Autodesk Inventor part; units mm, degrees
ref_plane "YZ Plane" through (0, 0, 0) normal (1, 0, 0) x (0, 1, 0)
ref_plane "XZ Plane" through (0, 0, 0) normal (0, 1, 0) x (-1, 0, 0)
ref_plane "XY Plane" through (0, 0, 0) normal (0, 0, 1) x (1, 0, 0)
sketch "Sketch1" plane through (0, 0, 0) normal (1, 0, 0) x (0, 1, 0)
  line L0 (-25, 30) -> (25, 30)
  line L1 (30, 25) -> (30, -25)
  line L2 (25, -30) -> (-25, -30)
  line L3 (-30, -25) -> (-30, 25)
  line L4 (-30, 30) -> (30, -30) construction
  line L5 (30, 30) -> (-30, -30) construction
  arc A0 (-25, 30) -> (-30, 25) centre (-25, 25) ccw
  arc A1 (-30, -25) -> (-25, -30) centre (-25, -25) ccw
  arc A2 (25, -30) -> (30, -25) centre (25, -25) ccw
  arc A3 (30, 25) -> (25, 30) centre (25, 25) ccw
  circle A4 centre (-20, 0) radius 4
  circle A5 centre (15, 15) radius 3.5
  circle A6 centre (15, -15) radius 3.5
  point P0 (0, 0)
  dimension "d0" = 60
  dimension "d1" = 60
  dimension "d6" = 5
  dimension "d7" = 8
  dimension "d10" = 15
  dimension "d11" = 30
  dimension "d12" = 15
  dimension "d13" = 7
  dimension "d14" = 35
extrude "Plate1" add sketch "Sketch1" along normal mid plane 5
sketch "Sketch2" plane through (2.5, 0, 0) normal (1, 0, 0) x (0, 0, -1)
  line L0 (-30, -30) -> (-10, -30)
  line L1 (-10, -30) -> (-10, 0)
  line L2 (-10, 0) -> (-30, 0)
  line L3 (-30, 0) -> (-30, -30)
  line L4 (30, -30) -> (10, -30)
  line L5 (10, -30) -> (10, 0)
  line L6 (10, 0) -> (30, 0)
  line L7 (30, 0) -> (30, -30)
  circle A0 centre (-15, 15) radius 3.5
  circle A1 centre (0, -20) radius 4
  line L8 (-30, -25) -> (-30, 25) construction
  point P0 (0, 0)
  dimension "d15" = 15
  dimension "d17" = 10
  dimension "d18" = 10
  dimension "d19" = 30
extrude "Cut1" cut sketch "Sketch2" against normal blind 5 contours L3 L2 L1 L0 | L4 L5 L6 L7
fillet "Corner Round1" radius 6 2 edges at (0, -30, 10) (0, -30, -10)
equation "\"d20\" = Thickness"
equation "\"d9\" = Thickness"
equation "\"BendRadius\" = Thickness"
equation "\"BendReliefWidth\" = Thickness"
equation "\"BendReliefDepth\" = 0.5 * Thickness"
equation "\"TransitionRadius\" = BendRadius"
equation "\"JacobiRadiusSize\" = BendRadius"
equation "\"GapSize\" = Thickness"
properties part number "HCMUTE-CDT23-BAT_CANG_BANG_TAI" material "Stainless Steel"
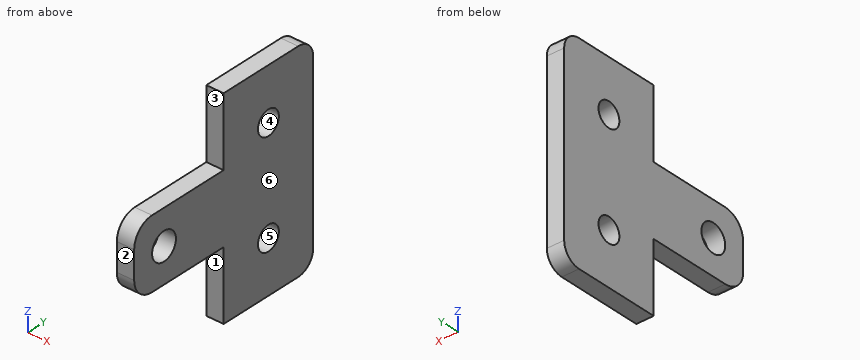
Could you check a few things on this model? Use its own coordinates, in mm. Face numbers are marked on the shaded views. A direction names the side the tool comes from. Round coordinates to 2 decimals unless told otherwise and drop trailing zeros. Write each loop counter-clockwise with the first axis right and the second up, starting at its lowest first coordinate (ties: lowest second). Pieces come first, ordered by that corner, then holes. Notation, with made-up numbers: (73.5, 45) -> (93.5, 45) arc R22 ccw to (93.5, 72) -> close; hole circle Ø1 at (32.25, 3). An arc over 180 degrees is marked (long way). Use a Markdown table: item, result.
1. Please list where these lines run through material, in increasing order: probe 1 along Z at (x, y) = (-1.2, 15); probe 2 along Z at (x, y) = (-0.5, -20); probe 3 along Y at (x, z) = (0.1, 24).
Answer key:
| item | result |
|---|---|
| probe 1 | z = -30 to -18.5, -11.5 to 11.5, 18.5 to 30 |
| probe 2 | z = -10 to -4, 4 to 10 |
| probe 3 | y = 0 to 30 |
2. If we section it at A-A (z = -15): List the corners of the cut face in (x, y) for me.
Answer key:
| item | result |
|---|---|
| outline | (-2.5, 0) -> (2.5, 0) -> (2.5, 11.5) -> (-2.5, 11.5) -> close; (-2.5, 18.5) -> (2.5, 18.5) -> (2.5, 30) -> (-2.5, 30) -> close |
3. Which directions (+Z, -Z, +X, -X, +Y, -Y) give clear straight access to the entire face, cutting with the end or side of a thin tool? Please do the marked faces 1 and 2.
Answer key:
| item | result |
|---|---|
| face 1 | -Z, +X, -X, -Y |
| face 2 | +Z, -Z, +X, -X, -Y |
4. If we section it at C-C (x = -0.9): List the corners of the cut face in (y, z) for me, then the cut area to 3 significant figures.
Answer key:
| item | result |
|---|---|
| outline | (-30, -4) arc R6 ccw to (-24, -10) -> (0, -10) -> (0, -30) -> (25, -30) arc R5 ccw to (30, -25) -> (30, 25) arc R5 ccw to (25, 30) -> (0, 30) -> (0, 10) -> (-24, 10) arc R6 ccw to (-30, 4) -> close; hole circle Ø8 at (-20, 0); hole circle Ø7 at (15, -15); hole circle Ø7 at (15, 15) |
| area | 2,250 mm^2 |
5. For pin 1 Ø6.5 at (y, z) = (15, -15) entering from +X; pin 2 Ø2.5 at (x, y) = (-0.5, -7) entering from +Z; pin 3 Ø1.5 at (x, z) = (0, 15.5) entering from -Y, each with a flat end and sliding along its axis, tell me the tip position at first contact or that it passes through.
Answer key:
| item | result |
|---|---|
| pin 1 | passes through |
| pin 2 | stops at z = 10 |
| pin 3 | stops at y = 0 |
6. We'd pull the mould along Y, two halves only. Please class the marked faces 3, 4, 5 and 6: +Y half, -Y half, draft (parallel to the pull), parting line (faces both ways), or undercut.
Answer key:
| item | result |
|---|---|
| face 3 | -Y half |
| face 4 | undercut |
| face 5 | undercut |
| face 6 | draft |
7. If we section it at B-B (y = -20): List the corners of the cut face in (x, z) for me, then the cut area to 3 significant figures.
Answer key:
| item | result |
|---|---|
| outline | (-2.5, -10) -> (2.5, -10) -> (2.5, -4) -> (-2.5, -4) -> close; (-2.5, 4) -> (2.5, 4) -> (2.5, 10) -> (-2.5, 10) -> close |
| area | 60.0 mm^2 |
8. If we section it at D-D (y = 15): List the corners of the cut face in (x, z) for me, then the cut area to 3 significant figures.
Answer key:
| item | result |
|---|---|
| outline | (-2.5, -30) -> (2.5, -30) -> (2.5, -18.5) -> (-2.5, -18.5) -> close; (-2.5, -11.5) -> (2.5, -11.5) -> (2.5, 11.5) -> (-2.5, 11.5) -> close; (-2.5, 18.5) -> (2.5, 18.5) -> (2.5, 30) -> (-2.5, 30) -> close |
| area | 230 mm^2 |
